Build history of the part. All positions in model axes, mm. A direction names the side the tool comes from. Coordinates: 2 decimals unless noted, no trailing zeros. Order: outer loops, then holes, each group sorted by start corner. A loop starts at its lowest first (then second) coordinate and runs counter-clockwise, first axis right, second up. Notation, with made-up numbers: (53.25, 68.5) - (82.25, 68.5) arc R10 ccw to (82.25, 84.5) - close; hole circle Ø10 at (51, -11). An arc over 180 degrees is marked (long way). Write each question's results on one line, items separated by ' | '. Start each with the question number.
from build123d import *

# Parameters (mm, degrees)
F2_W     = 5
F2_H     = 3
F3_DEPTH = 53.1


with BuildPart() as f1:
    # F0 (on Front) → F1 (revolve)
    with BuildSketch(Plane.XZ):
        with BuildLine():
            Line((0, -10), (-42, -10))
            Line((-42, -10), (-42, -20))
            Line((-42, -20), (-32, -20))
            ThreePointArc((-32, -20), (-28.464466, -21.464466), (-27, -25))
            Line((-27, -25), (-27, -43))
            Line((-27, -43), (-41.209174, -58.097248))
            ThreePointArc((-41.209174, -58.097248), (-42.82531, -65.141873), (-37.473933, -70))
            Line((-37.473933, -70), (-31.5, -70))
            Line((-31.5, -70), (-36, -63))
            Line((-36, -63), (-6, -63))
            Line((-6, -63), (-10.5, -70))
            Line((-10.5, -70), (-4.526067, -70))
            ThreePointArc((-4.526067, -70), (0.82531, -65.141873), (-0.790826, -58.097248))
            Line((-0.790826, -58.097248), (-15, -43))
            Line((-15, -43), (-15, -25))
            ThreePointArc((-15, -25), (-13.535534, -21.464466), (-10, -20))
            Line((-10, -20), (0, -20))
            Line((0, -20), (0, -10))
        make_face()
    revolve(axis=Axis((-21, 0, 0), (-1, 0, 0)))

    # F2 (on Right) → F3 (cut)
    with BuildSketch(Plane.YZ):
        with Locations((0, -11.075807)):
            Rectangle(F2_W, F2_H)
    extrude(amount=-F3_DEPTH, mode=Mode.SUBTRACT)


solid = f1.part
Item 1: Flat gauge pins, fed straight in: P1, Ø3, axis at y = -54, z = 24, coming from the +X side; P2, Ø2, axis at x = -33, z = 30, coming from the +Y side; P3, Ø3, axis at x = -31, z = -11, coming from the +Y side. Where does each tip first touch, or does it go through?
Item 2: Slice it at B-B (x = -8). Write the cut outline in (y, z) (1 decimal).
Item 3: Probe probe 1 along Y at (x, z) = (-26, 0); probe 2 along Z at (x, y) = (-30, 0); probe 3 along Z at (x, y) = (-19, 0). List the from-to ranges inside material, lowest first.
Item 4: Pull direction X, two halves, no side cores. Call faces 1 (the conical face through (-14.3, 42.7, 9.5)), 2 (the conical face through (-35.78, -62.8, 8.25)), 3 (the cylindrical face through (-20.79, -62.464, 8.201)), 4 (the flat face through (-42, -9, -5)): released by +X, released by -X, zero draft, split by the parting line, or undercut.
Item 5: Which spindle directions (+Z, -Z, +X, -X, +Y, -Y) get a long thin tool onto all of the face, cutting with end or side? Do faces 5 (the flat face through (-21, 0, -12.576)), 6 (the flat face through (-27, 19, 19)), 7 (the conical face through (-6.28, -42.87, 46.76)), 8 (the flat face through (-15, 19, -19)). Say none if no direction does.
Item 6: Slice it at A-A (x = -22). Write the cut outline in (y, z).
Resolved:
1) P1: x = 0.74 | P2: y = 63.71 | P3: y = 69.34
2) outline: circle Ø140 at (0, 0); circle Ø126 at (0, 0); circle Ø40 at (0, 0); hole circle Ø132.2 at (0, 0); hole circle Ø100.9 at (0, 0); hole (-2.5, -12.6) - (2.5, -12.6) - (2.5, -9.7) arc R10 ccw (long way) to (-2.5, -9.7) - close
3) probe 1: -63 to -10, 10 to 63 | probe 2: -63 to -46.19, -20.42 to -12.58, 10 to 20.42, 46.19 to 63 | probe 3: -63 to -12.58, 10 to 63
4) face 1: released by +X | face 2: undercut | face 3: undercut | face 4: released by -X
5) face 5: +X, -X | face 6: -X | face 7: none | face 8: +X
6) outline: circle Ø126 at (0, 0); hole (-2.5, -12.58) - (2.5, -12.58) - (2.5, -9.68) arc R10 ccw (long way) to (-2.5, -9.68) - close
